The listing builds one solid part. Answer for the finished solid, in the listing's coordinates (mm). Face numbers are marked on the shaded views. A direction names the side the tool comes from. Give positions to 0.01 mm unless a question says otherwise; leave off trailing zeros. Loops run counter-clockwise (first coordinate to the right, second up) from the corner with the lowest first, then second, coordinate; pieces in that order, holes last. Notation, with made-up numbers: M 73.5,35.25 L 78.5,35.25 A9 cw 78.5,45.25 Z; hole C 78.5,47.25 d11. An arc over 180 degrees is marked long. Use one line per item in the form item = value. Start each with the question number.
1. Straight lines are drawn through the part: line 1 (Z direction, x = 7.5, y = -1.3); line 2 (X direction, y = -2.3, z = 11.25); line 3 (X direction, y = -0.15, z = 12.25). For each, find the intervals that lie inside material, in ascending order. Write a range as from..to.
2. The part is cut by section C-C (y = -3.2). Write down the section's boundary in (x, z), and give its area (3 significant figures).
3. The part is cut by section D-D (z = 9.5). Write down the section's boundary in (x, y).
4. The mould has two halves that part along Z. Classify the marked faces 1, 2 and 3: released by +Z, released by -Z, zero draft, split by the parting line, or undercut.
5. The part is cut by section A-A (y = -1.1). Write down the section's boundary in (x, z), and give its area (3 significant figures).
6. The part is cut by section B-B (x = 27.5). Write down the section's boundary in (y, z).
7. For the marked faces 4 and 5, determine the directions among +Z, -Z, +X, -X, +Y, -Y from which every point of the face is accessible in a straight line to the end or side of a thin tool.
from build123d import *

# Parameters (mm, degrees)
SKETCH002_R      = 2.5
EXTRUDE002_DEPTH = 5
EXTRUDE001_DEPTH = 20
EXTRUDE_DEPTH    = 5


with BuildPart() as extrude002:
    # Sketch002 (on Cut) → Extrude002 (new body)
    with BuildSketch(Plane.XZ):
        with Locations((27.5, 10)):
            Circle(SKETCH002_R)
        with Locations((7.5, 10)):
            Circle(SKETCH002_R)
    extrude(amount=EXTRUDE002_DEPTH)


with BuildPart() as extrude001:
    # Sketch001 (on Extrude) → Extrude001 (new body)
    with BuildSketch(Plane.XY):
        Polygon((15.5, 0), (17.5, -2), (19.5, 0), align=None)
    extrude(amount=EXTRUDE001_DEPTH)


with BuildPart() as cut001:
    # Sketch → Extrude (new body)
    with BuildSketch(Plane.XZ):
        Polygon((0, 10), (5, 0), (30, 0), (35, 10), (35, 20), (0, 20), align=None)
    extrude(amount=EXTRUDE_DEPTH)

    # Cut: cut Extrude001
    add(extrude001.part, mode=Mode.SUBTRACT)

    # Cut001: cut Extrude002
    add(extrude002.part, mode=Mode.SUBTRACT)


solid = cut001.part
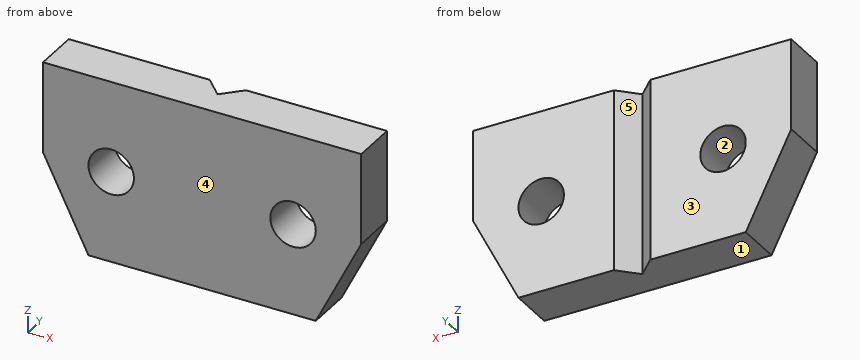
Derived:
q1.line_1 = 0..7.5, 12.5..20
q1.line_2 = 0..5.33, 9.67..25.33, 29.67..35
q1.line_3 = 0..6.41, 8.59..15.65, 19.35..26.41, 28.59..35
q2.outline = M 0,10 L 5,0 L 30,0 L 35,10 L 35,20 L 0,20 Z; hole C 7.5,10 d5; hole C 27.5,10 d5
q2.area = 611 mm2
q3.outline = M 0.25,-5 L 5.05,-5 L 5.05,0 L 0.25,0 Z; M 9.95,-5 L 25.05,-5 L 25.05,0 L 19.5,0 L 17.5,-2 L 15.5,0 L 9.95,0 Z; M 29.95,-5 L 34.75,-5 L 34.75,0 L 29.95,0 Z
q4.face_1 = released by -Z
q4.face_2 = undercut
q4.face_3 = zero draft
q5.outline = M 0,10 L 5,0 L 16.6,0 L 16.6,20 L 0,20 Z; M 18.4,0 L 30,0 L 35,10 L 35,20 L 18.4,20 Z; hole C 7.5,10 d5; hole C 27.5,10 d5
q5.area = 575 mm2
q6.outline = M -5,0 L 0,0 L 0,7.5 L -5,7.5 Z; M -5,12.5 L 0,12.5 L 0,20 L -5,20 Z
q7.face_4 = +Z, -Z, +X, -X, -Y
q7.face_5 = +Z, -Z, +Y
